Build history of the part. All positions in model axes, mm. Face numbers are marked on the shaded views. Round coordinates to 2 decimals unless told otherwise and drop trailing zeros. Order: outer loops, then holes, each group sorted by start corner. A loop starts at its lowest first (then second) coordinate and runs counter-clockwise, first axis right, second up. Notation, with made-up numbers: (35.25, 18) - (40.25, 18) arc R25 cw to (40.25, 37) - close; hole circle Ø8 at (68.25, -27.75). An arc over 180 degrees is marked (long way). One line per question, with ' | ' between items. Start each with the question number.
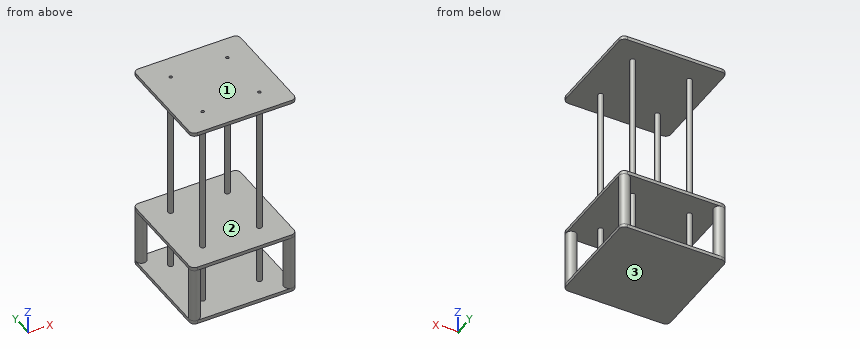
from build123d import *

# Parameters (mm, degrees)
ESQUISSE1_W             = 305
ESQUISSE1_H             = 305
BOSS_EXTRU_1_DEPTH      = 10
ESQUISSE2_R             = 15
BOSS_EXTRU_2_DEPTH      = 160
ESQUISSE3_W             = 305
ESQUISSE3_H             = 305
BOSS_EXTRU_3_DEPTH      = 10
ESQUISSE4_R             = 7.5
ENL_V_MAT_EXTRU_1_DEPTH = 281.913687812
BOSS_EXTRU_4_START      = -600
ESQUISSE5_R             = 7.5
BOSS_EXTRU_4_DEPTH      = 600
ESQUISSE7_W             = 305
ESQUISSE7_H             = 305
BOSS_EXTRU_5_DEPTH      = 10
D_GAGEMENT_M81_D        = 9
D_GAGEMENT_M81_DEPTH    = 10
D_GAGEMENT_M81_TIP      = 2.703872786
CONG_1_R                = 15


with BuildPart() as part:
    # Esquisse1 → Boss.-Extru.1 (new body)
    with BuildSketch(Plane.XY):
        Rectangle(ESQUISSE1_W, ESQUISSE1_H)
    extrude(amount=BOSS_EXTRU_1_DEPTH)

    # Esquisse2 → Boss.-Extru.2 (add)
    with BuildSketch(Plane.XY.offset(10)):
        with Locations((137.5, 137.5)):
            Circle(ESQUISSE2_R)
        with Locations((137.5, -137.5)):
            Circle(ESQUISSE2_R)
        with Locations(Location((-137.5, -137.5, 0), (0, 0, 180))):
            Circle(ESQUISSE2_R)
        with Locations(Location((-137.5, 137.5, 0), (0, 0, 180))):
            Circle(ESQUISSE2_R)
    extrude(amount=BOSS_EXTRU_2_DEPTH)

    # Esquisse3 → Boss.-Extru.3 (add)
    with BuildSketch(Plane.XY.offset(170)):
        Rectangle(ESQUISSE3_W, ESQUISSE3_H)
    extrude(amount=BOSS_EXTRU_3_DEPTH)

    # Esquisse4 → Enlèv. mat.-Extru.1 (cut, through all)
    with BuildSketch(Plane.XY.offset(180)):
        with Locations((82.5, -82.5)):
            Circle(ESQUISSE4_R)
        with Locations((-82.5, -82.5)):
            Circle(ESQUISSE4_R)
        with Locations((82.5, 82.5)):
            Circle(ESQUISSE4_R)
        with Locations((-82.5, 82.5)):
            Circle(ESQUISSE4_R)
    extrude(amount=-ENL_V_MAT_EXTRU_1_DEPTH, mode=Mode.SUBTRACT)

    # Esquisse5 → Boss.-Extru.4 (add)
    with BuildSketch(Plane(origin=(0, 0, 0), x_dir=(-1, 0, 0), z_dir=(0, 0, -1)).offset(BOSS_EXTRU_4_START)):
        with Locations((-82.5, 82.5)):
            Circle(ESQUISSE5_R)
        with Locations((82.5, 82.5)):
            Circle(ESQUISSE5_R)
        with Locations((82.5, -82.5)):
            Circle(ESQUISSE5_R)
        with Locations((-82.5, -82.5)):
            Circle(ESQUISSE5_R)
    extrude(amount=BOSS_EXTRU_4_DEPTH)

    # Esquisse7 → Boss.-Extru.5 (add)
    with BuildSketch(Plane.XY.offset(600)):
        Rectangle(ESQUISSE7_W, ESQUISSE7_H)
    extrude(amount=BOSS_EXTRU_5_DEPTH)

    # Dégagement M81
    with Locations(Plane(origin=(82.5, -82.5, 610), x_dir=(1, 0, 0), z_dir=(0, 0, 1))):
        with Locations((0, 0), (0, 165), (-165, 165), (-165, 0)):
            Hole(D_GAGEMENT_M81_D / 2, depth=D_GAGEMENT_M81_DEPTH)
            with Locations((0, 0, -(D_GAGEMENT_M81_DEPTH + D_GAGEMENT_M81_TIP / 2))):  # 118° drill point
                Cone(0, D_GAGEMENT_M81_D / 2, D_GAGEMENT_M81_TIP, mode=Mode.SUBTRACT)

    # Congé1
    cong_1_edges = [part.edges().sort_by_distance(p)[0] for p in [
        (-152.5, 152.5, 605),
        (-152.5, 152.5, 175),
        (-152.5, 152.5, 5),
        (-152.5, -152.5, 5),
        (-152.5, -152.5, 175),
        (-152.5, -152.5, 605),
        (152.5, -152.5, 605),
        (152.5, -152.5, 175),
        (152.5, -152.5, 5),
        (152.5, 152.5, 5),
        (152.5, 152.5, 175),
        (152.5, 152.5, 605),
    ]]
    fillet(cong_1_edges, radius=CONG_1_R - 0.0001)  # a hair under: the kernel refuses the full size


solid = part.part
Item 1: Wall check: line 1 along Y through (x, z) = (-82.5, 605.5); line 2 along Z through (x, y) = (-1, 76); line 3 along X through (y, z) = (-82, 606). Give the ranges that are in metal, low to high. Write a range as [from, to].
Item 2: Pull direction Z, two halves, no side cores. Call the marked faces 1, 2 and 3: released by +Z, released by -Z, zero draft, split by the parting line, or undercut.
Item 3: Slice it at A-A (y = -64). Write the cut outline in (x, z).
Item 4: Slice it at C-C (z = 216.5). Write the cut outline in (x, y), plus the area to 3 significant figures.
Item 5: Pin check, flat tips, straight feed: pin 1 (4 mm diameter, centred on y = -74.5, z = 198.5, fed in from +X); pin 2 (5 mm diameter, centred on x = 71.5, z = 406, fed in from +Y). Stop position of each tip, or through.
A:
1) line 1: [-152.5, -87], [-78, 78], [87, 152.5] | line 2: [0, 10], [170, 180], [600, 610] | line 3: [-152.5, -86.97], [-78.03, 78.03], [86.97, 152.5]
2) face 1: released by +Z | face 2: undercut | face 3: released by -Z
3) outline: (-152.5, 0) - (152.5, 0) - (152.5, 10) - (-152.5, 10) - close; (-152.5, 170) - (152.5, 170) - (152.5, 180) - (-152.5, 180) - close; (-152.5, 600) - (152.5, 600) - (152.5, 610) - (-152.5, 610) - close
4) outline: circle Ø15 at (-82.5, -82.5); circle Ø15 at (-82.5, 82.5); circle Ø15 at (82.5, -82.5); circle Ø15 at (82.5, 82.5) | area: 707 mm^2
5) pin 1: x = 87 | pin 2: through
